For this review, take the finished solid that the model builds, in its own axes (mm). A direction names the side the tool comes from. Give positions to 0.01 mm unless a question says otherwise; leave off trailing zeros. Loops run counter-clockwise (first coordinate to the right, second up) from the corner with the lowest first, then second, coordinate; pieces in that order, holes last.
```python
from build123d import *

# Parameters (mm, degrees)
BOSS_EXTRUDE1_DEPTH = 5
TAP1_D              = 4.134


with BuildPart() as part:
    # Sketch1 → Boss-Extrude1 (new, symmetric)
    with BuildSketch(Plane.XY):
        with BuildLine():
            Line((-4.1, 2.743829885), (-4.1, -2.743829885))
            ThreePointArc((-4.1, -2.743829885), (-4.06610325, -2.882354469), (-3.972072931, -2.989575498))
            Line((-3.972072931, -2.989575498), (-1.159973062, -4.958629024))
            ThreePointArc((-1.159973062, -4.958629024), (-0.923130974, -4.974152475), (-0.8, -4.771238909))
            Line((-0.8, -4.771238909), (-0.8, -2.9))
            Line((-0.8, -2.9), (-0.2, -2.9))
            ThreePointArc((-0.2, -2.9), (-0.058578644, -2.841421356), (0, -2.7))
            Line((0, -2.7), (0, 2.7))
            ThreePointArc((0, 2.7), (-0.058578644, 2.841421356), (-0.2, 2.9))
            Line((-0.2, 2.9), (-0.8, 2.9))
            Line((-0.8, 2.9), (-0.8, 4.771238909))
            ThreePointArc((-0.8, 4.771238909), (-0.923130974, 4.974152475), (-1.159973062, 4.958629024))
            Line((-1.159973062, 4.958629024), (-3.972072931, 2.989575498))
            ThreePointArc((-3.972072931, 2.989575498), (-4.06610325, 2.882354469), (-4.1, 2.743829885))
        make_face()
    extrude(amount=BOSS_EXTRUDE1_DEPTH, both=True)

    # Tap1 (through all)
    with Locations(Plane(origin=(0, 0, 0), x_dir=(0, 0, -1), z_dir=(1, 0, 0))):
        with Locations((0, 0)):
            Hole(TAP1_D / 2)


solid = part.part
```
Item 1: Take a section at B-B on y = 0. Give the boundary of the cut face in (x, z), and give its area (3 significant figures).
Answer:
outline: (-4.1, -5) - (0, -5) - (0, -2.07) - (-4.1, -2.07) - close; (-4.1, 2.07) - (0, 2.07) - (0, 5) - (-4.1, 5) - close
area: 24.1 mm2
Item 2: For L1, parallel to Y at x = -2.95, z = 0; L2, parallel to Z at x = -1.75, y = 1.75; L3, parallel to Y at x = -2.1, z = 0, list the stretches that pass through material, from the lowest coordinate up.
Answer:
L1: y = -3.71 to -2.07, 2.07 to 3.71
L2: z = -5 to -1.1, 1.1 to 5
L3: y = -4.3 to -2.07, 2.07 to 4.3
Item 3: Take a section at C-C on x = -2.8. Give the boundary of the cut face in (y, z), and give its area (3 significant figures).
Answer:
outline: (-3.81, -5) - (3.81, -5) - (3.81, 5) - (-3.81, 5) - close; hole circle Ø4.13 at (0, 0)
area: 62.8 mm2
Item 4: Clearance check with flat-ended pins moving along their axes: pin 1 Ø0.9 at (y, z) = (3.5, 0.5) entering from +X; pin 2 Ø1 at (x, z) = (-3, -0.5) entering from +Y; pin 3 Ø0.5 at (x, z) = (-0.5, -0.5) entering from -Y; pin 4 Ø3.5 at (y, z) = (0, 0) entering from -X. State where each tip first meets the part, or that it passes through.
Answer:
pin 1: stops at x = -0.8
pin 2: stops at y = 4.02
pin 3: stops at y = -2.9
pin 4: passes through
Item 5: Tool access review of faces 4 (the flat face through (-0.8, -4, 0)), 5 (the flat face through (-0.8, 4, 0)), 6 (the flat face through (-2.586, -3.96, 0.07)): name each direction out of +Z, -Z, +X, -X, +Y, -Y from which nothing blocks a thin tool from reaching the whole face with its end or side.
Answer:
face 4: +Z, -Z, +X, -Y
face 5: +Z, -Z, +X, +Y
face 6: +Z, -Z, -X, -Y
Item 6: Take a section at A-A on z = 0. Give the boundary of the cut face in (x, y), and give its area (3 significant figures).
Answer:
outline: (-4.1, -2.74) arc R0.3 ccw to (-3.97, -2.99) - (-1.16, -4.96) arc R0.23 ccw to (-0.8, -4.77) - (-0.8, -2.9) - (-0.2, -2.9) arc R0.2 ccw to (0, -2.7) - (0, -2.07) - (-4.1, -2.07) - close; (-4.1, 2.07) - (0, 2.07) - (0, 2.7) arc R0.2 ccw to (-0.2, 2.9) - (-0.8, 2.9) - (-0.8, 4.77) arc R0.23 ccw to (-1.16, 4.96) - (-3.97, 2.99) arc R0.3 ccw to (-4.1, 2.74) - close
area: 14.3 mm2
Item 7: The part is to be moulded in two halves that separate along Y. For faces 1 (the cylindrical face through (-2.08, -1.26, -1.64)), 2 (the flat face through (0, -2, 1)), 3 (the flat face through (-2.546, 3.988, 0.07)), say which applies: released by +Y, released by -Y, zero draft, split by the parting line, or undercut.
Answer:
face 1: undercut
face 2: zero draft
face 3: released by +Y
Item 8: Take a section at D-D on z = 3.5. Give the boundary of the cut face in (x, y).
Answer:
outline: (-4.1, -2.74) arc R0.3 ccw to (-3.97, -2.99) - (-1.16, -4.96) arc R0.23 ccw to (-0.8, -4.77) - (-0.8, -2.9) - (-0.2, -2.9) arc R0.2 ccw to (0, -2.7) - (0, 2.7) arc R0.2 ccw to (-0.2, 2.9) - (-0.8, 2.9) - (-0.8, 4.77) arc R0.23 ccw to (-1.16, 4.96) - (-3.97, 2.99) arc R0.3 ccw to (-4.1, 2.74) - close
